For this review, take the finished solid that the model builds, in its own axes (mm). A direction names the side the tool comes from. Coordinates: 2 decimals unless noted, no trailing zeros. Loops run counter-clockwise (first coordinate to the right, second up) from the corner with the lowest first, then second, coordinate; pieces in that order, holes last. Notation, with made-up numbers: (-33.75, 21) -> (-3.75, 21) arc R21 ccw to (-3.75, 60) -> close; hole circle Ø4 at (-4.5, 67). An arc over 180 degrees is marked (long way). Answer in a Markdown table with one row per item.
from build123d import *

# Parameters (mm, degrees)
F3_START = -1.34776
F2_W     = 11.6723957472
F2_H     = 7.4633890763
F3_DEPTH = 23.65224
F5_START = 0.96875
F4_W     = 10.800289805
F4_H     = 7.1797380224
F5_DEPTH = 7.09642
F6_R     = 1.95
F7_DEPTH = 12.5


with BuildPart() as f1:
    # F0 (on Front) → F1 (revolve)
    with BuildSketch(Plane.XZ):
        with BuildLine():
            Line((-7.0006786053, 12.4883897992), (-5.3249788856, 8.0614940048))
            Line((-5.3249788856, 8.0614940048), (-5.3249788856, -12.3409103399))
            Line((-5.3249788856, -12.3409103399), (-6.6749788856, -12.3409103399))
            Line((-6.6749788856, -12.3409103399), (-6.6749788856, -14.3409103399))
            Line((-6.6749788856, -14.3409103399), (-5.3249788856, -14.3409103399))
            Line((-5.3249788856, -14.3409103399), (-5.3249788856, -25.5409103399))
            ThreePointArc((-5.3249788856, -25.5409103399), (-4.9149283792, -26.5308598336), (-3.9249788856, -26.9409103399))
            Line((-3.9249788856, -26.9409103399), (-3.0749788856, -26.9409103399))
            Line((-3.0749788856, -26.9409103399), (-3.0749788856, 10.274941902))
            ThreePointArc((-3.0749788856, 10.274941902), (-4.5898110963, 11.7897741127), (-3.0749788856, 13.3046063234))
            Line((-3.0749788856, 13.3046063234), (-3.0749788856, 14.8147279002))
            Line((-3.0749788856, 14.8147279002), (-5.2641126534, 14.8147279002))
            Line((-5.2641126534, 14.8147279002), (-7.0006786053, 12.4883897992))
        make_face()
    revolve(axis=Axis((-3.0749788856, 0, -4.5506457565), (0, 0, 1)))

    # F2 (on Front) → F3 (cut)
    with BuildSketch(Plane.XZ.offset(F3_START)):
        with Locations((-2.7008608449, 11.793188543)):
            Rectangle(F2_W, F2_H)
    extrude(amount=-F3_DEPTH, mode=Mode.SUBTRACT)

    # F4 (on Front) → F5 (cut)
    with BuildSketch(Plane.XZ.offset(F5_START)):
        with Locations((-3.5045757541, 11.651363016)):
            Rectangle(F4_W, F4_H)
    extrude(amount=F5_DEPTH, mode=Mode.SUBTRACT)

    # F6 (on face) → F7 (cut, symmetric)
    with BuildSketch(Plane.XZ.offset(0.96875)):
        with Locations((-3.0749788856, 11.7897741127)):
            Circle(F6_R)
    extrude(amount=F7_DEPTH, both=True, mode=Mode.SUBTRACT)


solid = f1.part
Item 1: The part is to be moulded in two halves that separate along Z. For faces 4 (the cylindrical face through (-3.498, 0.173, 9.886)), 5 (the flat face through (-3.1, -1.5, 8.061)), 6 (the flat face through (-1, 1.348, 13)), say which applies: +Z half, -Z half, draft (parallel to the pull), parting line (faces both ways), or undercut.
Worked answers:
| item | result |
|---|---|
| face 4 | undercut |
| face 5 | +Z half |
| face 6 | draft |
Item 2: For L1, parallel to Z at x = -2.75, y = 1.25; L2, parallel to Y at x = -1, z = 12.5; L3, parallel to Z at x = -4, y = 2.5, list the stretches that pass through material, from the lowest coordinate up.
Worked answers:
| item | result |
|---|---|
| L1 | -26.87 to 9.87, 13.71 to 14.81 |
| L2 | -0.97 to 1.35 |
| L3 | -14.34 to -12.34 |
Item 3: Take a section at A-A, the plane z = -18. State the section outline as (x, y) points, and give its area (3 significant figures).
Worked answers:
| item | result |
|---|---|
| outline | circle Ø4.5 at (-3.07, 0) |
| area | 15.9 mm² |
Item 4: For faces 1 (the flat face through (-5, 2, -12.341)), 2 (the conical face through (-0.197, 0.263, 9.752)), 3 (the cylindrical face through (-0.827, -0.099, -20.019)), list the 3-axis set-ups (+Z, -Z, +X, -X, +Y, -Y) from which the entire face can be reached by the end or side of a thin tool; tool diameter is ignored.
Worked answers:
| item | result |
|---|---|
| face 1 | none |
| face 2 | +X |
| face 3 | -Z |
Item 5: Insertion check: pin 1 (3 mm diameter, centred on y = 2, z = 7, fed in from -X); pin 2 (0.6 mm diameter, centred on x = -2.5, y = -1.5, fed in from +Z). Each pin has a flat end and moves straight along its axis. Give the tip position at first contact, or say it passes through.
Worked answers:
| item | result |
|---|---|
| pin 1 | x = -5.27 |
| pin 2 | z = 8.06 |
